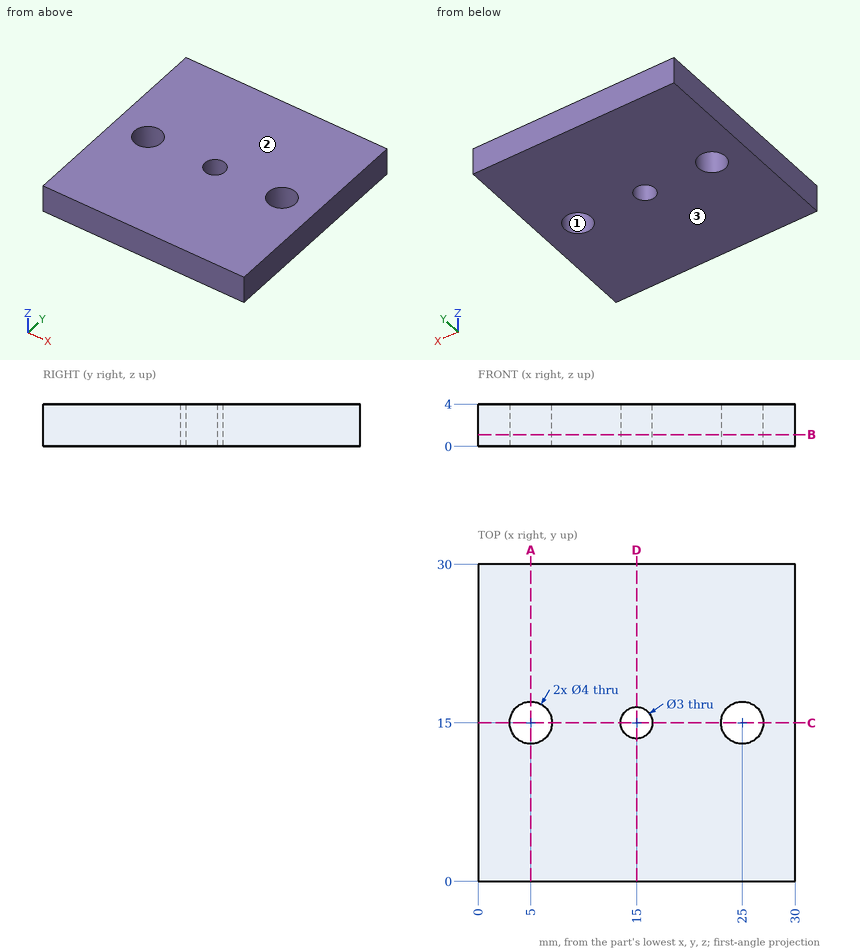
Source: three-view drawing plus pictorial views. Frame: mm from the lowest corner of the part. Round coordinates to 2 decimals unless told otherwise and drop trailing zeros. Loops run counter-clockwise (first coordinate to the right, second up) from the corner with the lowest first, then second, coordinate; pieces in that order, holes last. Notation, with made-up numbers: M -12.5,10 L 7.5,10 A24 ccw 7.5,35 Z; hole C 47,22 d11. An arc over 180 degrees is marked long. Answer as CSV lines item,"result".
Q1. Line query: line 1 along X through (y, z) = (15, 0.8); line 2 along Y through (x, z) = (15, 3.05); line 3 along Y through (x, z) = (25, 2.3). Output: solid intervals per line, ascending.
Verdict:
line 1,"x = 0 to 3, 7 to 13.5, 16.5 to 23, 27 to 30"
line 2,"y = 0 to 13.5, 16.5 to 30"
line 3,"y = 0 to 13, 17 to 30"
Q2. Cut plane B-B (z = 1.1). Return the cut outline in (x, y).
Verdict:
outline,"M 0,0 L 30,0 L 30,30 L 0,30 Z; hole C 5,15 d4; hole C 15,15 d3; hole C 25,15 d4"
Q3. Pull-direction query (Z, two-part tool) for the marked faces 1, 2 and 3; classes: +Z half, -Z half, draft (parallel to the pull), parting line (faces both ways), or undercut.
Verdict:
face 1,"draft"
face 2,"+Z half"
face 3,"-Z half"
Q4. Cut plane A-A (x = 5). Return the cut outline in (y, z).
Verdict:
outline,"M 0,0 L 13,0 L 13,4 L 0,4 Z; M 17,0 L 30,0 L 30,4 L 17,4 Z"
Q5. Cut plane C-C (y = 15). Return the cut outline in (x, z), plus the area to 3 significant figures.
Verdict:
outline,"M 0,0 L 3,0 L 3,4 L 0,4 Z; M 7,0 L 13.5,0 L 13.5,4 L 7,4 Z; M 16.5,0 L 23,0 L 23,4 L 16.5,4 Z; M 27,0 L 30,0 L 30,4 L 27,4 Z"
area,"76.0 mm^2"
Q6. Cut plane D-D (x = 15). Return the cut outline in (y, z).
Verdict:
outline,"M 0,0 L 13.5,0 L 13.5,4 L 0,4 Z; M 16.5,0 L 30,0 L 30,4 L 16.5,4 Z"
